Design review of the part built by this model. Coordinates are the model's own, in mm. Face numbers are marked on the shaded views. A direction names the side the tool comes from. Give positions to 0.01 mm unless a question says otherwise; leave off trailing zeros. Loops run counter-clockwise (first coordinate to the right, second up) from the corner with the lowest first, then second, coordinate; pieces in that order, holes last. Notation, with made-up numbers: (-21, 18.25) - (19, 18.25) arc R21 ccw to (19, 41.25) - close; hole circle Ø11 at (7, -20). An arc over 180 degrees is marked (long way). Write each question's results on one line, items separated by ' | '.
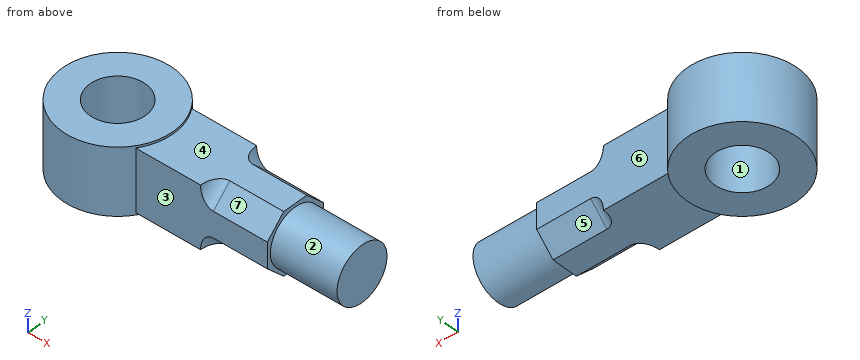
```python
from build123d import *

# Parameters (mm, degrees)
SKETCH1_R           = 25
SKETCH1_R_2         = 12.5
BOSS_EXTRUDE1_DEPTH = 30
BOSS_EXTRUDE2_DEPTH = 14
BOSS_EXTRUDE5_DEPTH = 30
FILLET6_R           = 5.75
FILLET7_R           = 5.75
FILLET8_R           = 5.75
FILLET9_R           = 5.75
SKETCH7_R           = 12.5
BOSS_EXTRUDE6_DEPTH = 30


with BuildPart() as part:
    # Sketch1 → Boss-Extrude1 (new body)
    with BuildSketch(Plane.XY):
        Circle(SKETCH1_R)
        Circle(SKETCH1_R_2, mode=Mode.SUBTRACT)
    extrude(amount=BOSS_EXTRUDE1_DEPTH)

    # Sketch2 → Boss-Extrude2 (add, symmetric)
    with BuildSketch(Plane(origin=(0, 0, 15), x_dir=(-1, 0, 0), z_dir=(0, 0, -1))):
        with BuildLine():
            ThreePointArc((-20.712315177, 14), (-25, 0), (-20.712315177, -14))
            Line((-20.712315177, -14), (-49.87018371, -14))
            Line((-49.87018371, -14), (-49.87018371, 14))
            Line((-49.87018371, 14), (-20.712315177, 14))
        make_face()
    extrude(amount=BOSS_EXTRUDE2_DEPTH, both=True)

    # Sketch6 → Boss-Extrude5 (add)
    with BuildSketch(Plane(origin=(49.87018371, 0, 0), x_dir=(0, 0, -1), z_dir=(1, 0, 0))):
        Polygon((-9.201010127, 14), (-20.798989873, 14), (-29, 5.798989873), (-29, -5.798989873), (-20.798989873, -14), (-9.201010127, -14), (-1, -5.798989873), (-1, 5.798989873), align=None)
    extrude(amount=BOSS_EXTRUDE5_DEPTH)

    # Fillet6
    fillet6_edges = [part.edges().sort_by_distance(p)[0] for p in [
        (49.87018371, 9.899494937, 24.899494937),
    ]]
    fillet(fillet6_edges, radius=FILLET6_R)

    # Fillet7
    fillet7_edges = [part.edges().sort_by_distance(p)[0] for p in [
        (49.87018371, 9.899494937, 5.100505063),
    ]]
    fillet(fillet7_edges, radius=FILLET7_R)

    # Fillet8
    fillet8_edges = [part.edges().sort_by_distance(p)[0] for p in [
        (49.87018371, -9.899494937, 24.899494937),
    ]]
    fillet(fillet8_edges, radius=FILLET8_R)

    # Fillet9
    fillet9_edges = [part.edges().sort_by_distance(p)[0] for p in [
        (49.87018371, -9.899494937, 5.100505063),
    ]]
    fillet(fillet9_edges, radius=FILLET9_R)

    # Sketch7 → Boss-Extrude6 (add)
    with BuildSketch(Plane(origin=(79.87018371, 0, 0), x_dir=(0, 0, -1), z_dir=(1, 0, 0))):
        with Locations((-15, 0)):
            Circle(SKETCH7_R)
    extrude(amount=BOSS_EXTRUDE6_DEPTH)


solid = part.part
```
Item 1: We need section D-D on z = 15. Give the boundary of the cut face in (x, y).
Output values:
outline: (20.71, -14) - (79.87, -14) - (79.87, -12.5) - (109.87, -12.5) - (109.87, 12.5) - (79.87, 12.5) - (79.87, 14) - (20.71, 14) arc R25 ccw (long way) to start; hole circle Ø25 at (0, 0)
Item 2: We need section C-C on x = 76. Give the boundary of the cut face in (y, z).
Output values:
outline: (-14, 9.2) - (-5.8, 1) - (5.8, 1) - (14, 9.2) - (14, 20.8) - (5.8, 29) - (-5.8, 29) - (-14, 20.8) - close
Item 3: Wall thickness on probe 1 along Y at (x, z) = (0, 22.75); probe 2 along Y at (x, z) = (39.5, 4); probe 3 along Z at (x, y) = (29, -5): over which ranges is each line inside the solid? List them lowest first.
Output values:
probe 1: y = -25 to -12.5, 12.5 to 25 | probe 2: y = -14 to 14 | probe 3: z = 1 to 29
Item 4: We need section B-B on x = 0. Give the boundary of the cut face in (y, z), then the cut area to 3 significant figures.
Output values:
outline: (-25, 0) - (-12.5, 0) - (-12.5, 30) - (-25, 30) - close; (12.5, 0) - (25, 0) - (25, 30) - (12.5, 30) - close | area: 750 mm²
Item 5: Tool access review of the marked faces 5, 6 and 7: name each direction out of +Z, -Z, +X, -X, +Y, -Y from which nothing blocks a thin tool from reaching the whole face with its end or side.
Output values:
face 5: -Z, +X, +Y | face 6: +Z, -Z, +X, +Y | face 7: +Z, +X, -Y
Item 6: We need section A-A on y = -4. Give the boundary of the cut face in (x, z), then the cut area to 3 significant figures.
Output values:
outline: (-24.68, 0) - (-11.84, 0) - (-11.84, 30) - (-24.68, 30) - close; (11.84, 0) - (24.68, 0) - (24.68, 1) - (79.87, 1) - (79.87, 3.16) - (109.87, 3.16) - (109.87, 26.84) - (79.87, 26.84) - (79.87, 29) - (24.68, 29) - (24.68, 30) - (11.84, 30) - close | area: 3,030 mm²
Item 7: Draft analysis for pull direction Y (two halves, no side actions). For the marked faces 1, 2, 3 and 4, state which applies: +Y half, -Y half, draft (parallel to the pull), parting line (faces both ways), or undercut.
Output values:
face 1: undercut | face 2: parting line | face 3: -Y half | face 4: draft
Item 8: Clearance check with flat-ended pins moving along their axes: P1, Ø5, axis at y = -13, z = 7, coming from the -X side; P2, Ø3, axis at x = 33, y = -9.5, coming from the -Z side; P3, Ø10, axis at x = 2.5, y = -3, coming from the -Z side; P4, Ø8.5, axis at x = 41, z = 21.5, coming from the -Y side. State where each tip first meets the part, or that it passes through.
Output values:
P1: stops at x = -22.69 | P2: stops at z = 1 | P3: passes through | P4: stops at y = -14
